Autodesk Inventor part; units mm, degrees
ref_plane "YZ Plane" through (0, 0, 0) normal (1, 0, 0) x (0, 1, 0)
ref_plane "XZ Plane" through (0, 0, 0) normal (0, 1, 0) x (-1, 0, 0)
ref_plane "XY Plane" through (0, 0, 0) normal (0, 0, 1) x (1, 0, 0)
sketch "Sketch34" plane through (0, 0, 0) normal (0, 0, 1) x (1, 0, 0)
  line L0 (0, 0) -> (30, 0)
  line L1 (30, 0) -> (30, -30)
  line L2 (30, -30) -> (0, -30)
  line L3 (0, -30) -> (0, 0)
  dimension "d112" = 30
  dimension "d113" = 30
extrude "Extrusion25" add sketch "Sketch34" against normal blind 10
sketch "Sketch35" plane through (30, -30, 0) normal (1, 0, 0) x (0, 0, -1)
  line L0 (0, 30) -> (10, 30)
  line L1 (0, 30) -> (30, 30)
  line L2 (30, 30) -> (30, 0)
  line L3 (30, 0) -> (0, 0)
  line L4 (0, 0) -> (0, 30)
  dimension "d116" = 30
  dimension "d117" = 30
extrude "Extrusion26" add sketch "Sketch35" against normal blind 10
sketch "Sketch37" plane through (30, -30, 0) normal (1, 0, 0) x (0, 0, -1)
  point P0 (0, 30)
sketch "Sketch38" plane through (30, -30, 0) normal (1, 0, 0) x (0, 0, -1)
  circle A0 centre (15, 15) radius 3
  point P0 (0, 30)
  dimension "d123" = 6
extrude "Extrusion28" cut sketch "Sketch38" against normal blind 10
sketch "Sketch39" plane through (30, -30, 0) normal (1, 0, 0) x (0, 0, -1)
  point P0 (0, 30)
sketch "Sketch43" plane through (20, -30, 0) normal (-1, 0, 0) x (0, 0, 1)
  circle A0 centre (-15, 15) radius 4.5
  point P0 (0, 30)
  dimension "d135" = 9
extrude "Extrusion32" cut sketch "Sketch43" against normal blind 5
sketch "Sketch44" plane through (0, 0, -10) normal (0, 0, -1) x (-1, 0, 0)
  circle A0 centre (-15, -15) radius 4.5
  point P0 (0, 0)
  dimension "d138" = 9
extrude "Extrusion33" cut sketch "Sketch44" against normal blind 5
sketch "Sketch45" plane through (0, 0, 0) normal (0, 0, 1) x (1, 0, 0)
  circle A0 centre (15, -15) radius 4.5
  circle A1 centre (15, -15) radius 3
  point P0 (0, 0)
  dimension "d141" = 6
extrude "Extrusion34" cut sketch "Sketch45" against normal blind 10 contours A1
properties part number "tunnel corner bracket_v02"
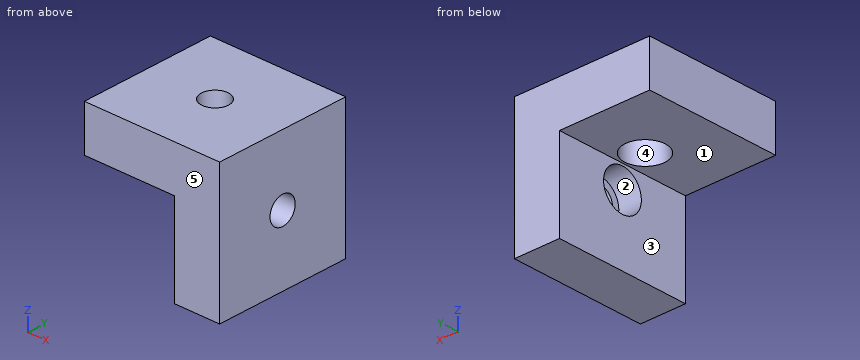
Can you work these out from the model? Positions are in its coordinate system, mm. Face numbers are marked on the shaded views. A direction names the side the tool comes from. Give positions to 0.01 mm unless a question says otherwise; leave off trailing zeros. Loops run counter-clockwise (first coordinate to the right, second up) from the corner with the lowest first, then second, coordinate; pieces in that order, holes last. Notation, with made-up numbers: (57, 6) - (111, 6) arc R15 ccw to (111, 19) - close; hole circle Ø2 at (-28.5, -3). An arc over 180 degrees is marked (long way). Answer as a JSON object with one key per item and string values.
Q1. Imagine slicing it at B-B on z = -15. Write out the boundary of the cut face in (x, y), plus the area to 3 significant figures.
Geometry says:
{"outline": "(20, -30) - (30, -30) - (30, -18) - (25, -18) - (25, -19.5) - (20, -19.5) - close; (20, -10.5) - (25, -10.5) - (25, -12) - (30, -12) - (30, 0) - (20, 0) - close", "area": "225 mm²"}
Q2. If we mould it in two halves opening along Z, with no side actions, what happens to the marked faces 1, 2 and 3? For each: pulls with the +Z half, pulls with the -Z half, needs draft (parallel to the pull), parting line crosses it, or undercut.
Geometry says:
{"face 1": "pulls with the -Z half", "face 2": "undercut", "face 3": "needs draft"}
Q3. Which directions (+Z, -Z, +X, -X, +Y, -Y) give clear straight access to the entire face, cutting with the end or side of a thin tool? Please do the marked faces 4 and 5.
Geometry says:
{"face 4": "-Z", "face 5": "+Z, -Z, +X, -X, -Y"}
Q4. Imagine slicing it at D-D on x = 27.75. Write out the boundary of the cut face in (y, z).
Geometry says:
{"outline": "(-30, -30) - (0, -30) - (0, 0) - (-30, 0) - close; hole circle Ø6 at (-15, -15)"}
Q5. Imagine slicing it at C-C on x = 15. Write out the boundary of the cut face in (y, z), plus the area to 3 significant figures.
Geometry says:
{"outline": "(-30, -10) - (-19.5, -10) - (-19.5, -5) - (-18, -5) - (-18, 0) - (-30, 0) - close; (-12, -5) - (-10.5, -5) - (-10.5, -10) - (0, -10) - (0, 0) - (-12, 0) - close", "area": "225 mm²"}
Q6. Imagine slicing it at A-A on y = -15. Write out the boundary of the cut face in (x, z), plus the area to 3 significant figures.
Geometry says:
{"outline": "(0, -10) - (10.5, -10) - (10.5, -5) - (12, -5) - (12, 0) - (0, 0) - close; (18, -5) - (19.5, -5) - (19.5, -10) - (20, -10) - (20, -10.5) - (25, -10.5) - (25, -12) - (30, -12) - (30, 0) - (18, 0) - close; (20, -30) - (30, -30) - (30, -18) - (25, -18) - (25, -19.5) - (20, -19.5) - close", "area": "350 mm²"}
Q7. If I drill on L1, parallel to Y at x = 15, z = -7.75; L2, parallel to Z at x = 13.5, y = -25.25; L3, parallel to X at y = -17.75, z = -21.5, over which ranges is the centre line in solid material (lowest first)?
Geometry says:
{"L1": "-30 to -19.5, -10.5 to 0", "L2": "-10 to 0", "L3": "20 to 30"}
Q8. Will these pins go through, and if not, where does the flat tip stop? P1, Ø2, axis at y = -4, z = -17.5, coming from the -X side; P2, Ø8, axis at x = 10, y = -3, coming from the -Z side; P3, Ø2.5, axis at y = -16.5, z = -16, coming from the -X side.
Geometry says:
{"P1": "x = 20", "P2": "z = -10", "P3": "x = 25"}
